CAD build for the part. Positions are in the model's coordinates, mm. A direction names the side the tool comes from. Coordinates: 2 decimals unless noted, no trailing zeros. Order: outer loops, then holes, each group sorted by start corner. A loop starts at its lowest first (then second) coordinate and runs counter-clockwise, first axis right, second up. Notation, with made-up numbers: (18.25, 56) - (26.25, 56) arc R15 ccw to (26.25, 74) - close; hole circle Ø9 at (-22.5, -16). An arc over 180 degrees is marked (long way). Use one line per item in the form item = value.
```python
from build123d import *

# Parameters (mm, degrees)
F0_W     = 30
F0_H     = 30
F1_DEPTH = 3
F2_R     = 10
F2_R_2   = 8
F3_DEPTH = 15
F5_DEPTH = 15


with BuildPart() as f1:
    # F0 (on Top) → F1 (new body)
    with BuildSketch(Plane.XY):
        Rectangle(F0_W, F0_H)
    extrude(amount=F1_DEPTH)

    # F2 (on face) → F3 (join)
    with BuildSketch(Plane.XY.offset(3)):
        Circle(F2_R)
        Circle(F2_R_2, mode=Mode.SUBTRACT)
    extrude(amount=F3_DEPTH)

    # F4 (on face) → F5 (cut, through all)
    with BuildSketch(Plane.XY.offset(18)):
        with BuildLine():
            Line((-4.495868, 6.617188), (-5.930406, 8.051726))
            ThreePointArc((-5.930406, 8.051726), (-7.071068, 7.071068), (-8.051726, 5.930406))
            Line((-8.051726, 5.930406), (-6.617188, 4.495868))
            ThreePointArc((-6.617188, 4.495868), (-5.656854, 5.656854), (-4.495868, 6.617188))
        make_face()
        with BuildLine():
            ThreePointArc((8.051726, 5.930406), (7.071068, 7.071068), (5.930406, 8.051726))
            Line((5.930406, 8.051726), (4.495868, 6.617188))
            ThreePointArc((4.495868, 6.617188), (5.656854, 5.656854), (6.617188, 4.495868))
            Line((6.617188, 4.495868), (8.051726, 5.930406))
        make_face()
        with BuildLine():
            ThreePointArc((5.930406, -8.051726), (7.071068, -7.071068), (8.051726, -5.930406))
            Line((8.051726, -5.930406), (6.617188, -4.495868))
            ThreePointArc((6.617188, -4.495868), (5.656854, -5.656854), (4.495868, -6.617188))
            Line((4.495868, -6.617188), (5.930406, -8.051726))
        make_face()
        with BuildLine():
            Line((-6.617188, -4.495868), (-8.051726, -5.930406))
            ThreePointArc((-8.051726, -5.930406), (-7.071068, -7.071068), (-5.930406, -8.051726))
            Line((-5.930406, -8.051726), (-4.495868, -6.617188))
            ThreePointArc((-4.495868, -6.617188), (-5.656854, -5.656854), (-6.617188, -4.495868))
        make_face()
    extrude(amount=-F5_DEPTH, mode=Mode.SUBTRACT)


solid = f1.part
```
Item 1: Drill centre lines: line 1 (Z direction, x = 13.75, y = -9.75); line 2 (X direction, y = -7.25, z = 16.5); line 3 (X direction, y = 2, z = 14.5). Where is each one in solid material? Low to high. Write a range as [from, to].
Derived:
line_1 = [0, 3]
line_2 = [-5.13, -3.38], [3.38, 5.13]
line_3 = [-9.8, -7.75], [7.75, 9.8]
Item 2: Cut at A-A, the plane z = 10.5. Write the cut outline in (x, y).
Derived:
outline = (-8.05, -5.93) - (-6.62, -4.5) arc R8 cw to (-6.62, 4.5) - (-8.05, 5.93) arc R10 ccw to start; (-5.93, -8.05) arc R10 ccw to (5.93, -8.05) - (4.5, -6.62) arc R8 cw to (-4.5, -6.62) - close; (-5.93, 8.05) - (-4.5, 6.62) arc R8 cw to (4.5, 6.62) - (5.93, 8.05) arc R10 ccw to start; (6.62, -4.5) - (8.05, -5.93) arc R10 ccw to (8.05, 5.93) - (6.62, 4.5) arc R8 cw to start
Item 3: Cut at B-B, the plane y = 0.25. Write the cut outline in (x, z), plus the area to 3 significant figures.
Derived:
outline = (-15, 0) - (15, 0) - (15, 3) - (10, 3) - (10, 18) - (8, 18) - (8, 3) - (-8, 3) - (-8, 18) - (-10, 18) - (-10, 3) - (-15, 3) - close
area = 150 mm²
Item 4: Two-plate mould, pull along Y, no slides. Class faces 5 (the face through (-5.22, -7.34, 10.6)), 6 (the face through (-7.34, 5.22, 10.6)), 7 (the face through (10, 0, 10)), 8 (the face through (15, 0, 1)): +Y half, -Y half, draft (parallel to the pull), parting line (faces both ways), or undercut.
Derived:
face_5 = undercut
face_6 = +Y half
face_7 = parting line
face_8 = draft
Item 5: Drop flat-ended pins along their axis: pin 1 (1 mm diameter, centred on x = 6.5, y = 10.5, fed in from +Z); pin 2 (8 mm diameter, centred on y = -9.5, z = 9, fed in from -X). Give the stop position or say it passes through.
Derived:
pin_1 = 3
pin_2 = -8.35
Item 6: 3-axis set-ups, long thin cutter, end or side, ignore diameter. For faces 1 (the face through (0, 8, 10)), 2 (the face through (7.32, 5.2, 10.6)), 3 (the face through (5.22, 7.34, 10.6)), 4 (the face through (0, -10, 10)): which of +Z, -Z, +X, -X, +Y, -Y reach the whole face in a straight line?
Derived:
face_1 = +Z
face_2 = +Z, +Y
face_3 = +Z, +X
face_4 = +Z, -Y
Item 7: Cut at D-D, the plane x = 2.5. Write the cut outline in (y, z).
Derived:
outline = (-15, 0) - (15, 0) - (15, 3) - (9.68, 3) - (9.68, 18) - (7.6, 18) - (7.6, 3) - (-7.6, 3) - (-7.6, 18) - (-9.68, 18) - (-9.68, 3) - (-15, 3) - close
Item 8: Cut at C-C, the plane x = 9.5. Write the cut outline in (y, z).
Derived:
outline = (-15, 0) - (15, 0) - (15, 3) - (3.12, 3) - (3.12, 18) - (-3.12, 18) - (-3.12, 3) - (-15, 3) - close
